Part print with two shaded views. Sizes in mm from the minimum x, y, z corner. A direction names the side the tool comes from. Coordinates: 2 decimals unless noted, no trailing zeros. Write each loop counter-clockwise with the first axis right and the second up, starting at its lowest first coordinate (ties: lowest second). Pieces come first, ordered by that corner, then holes.
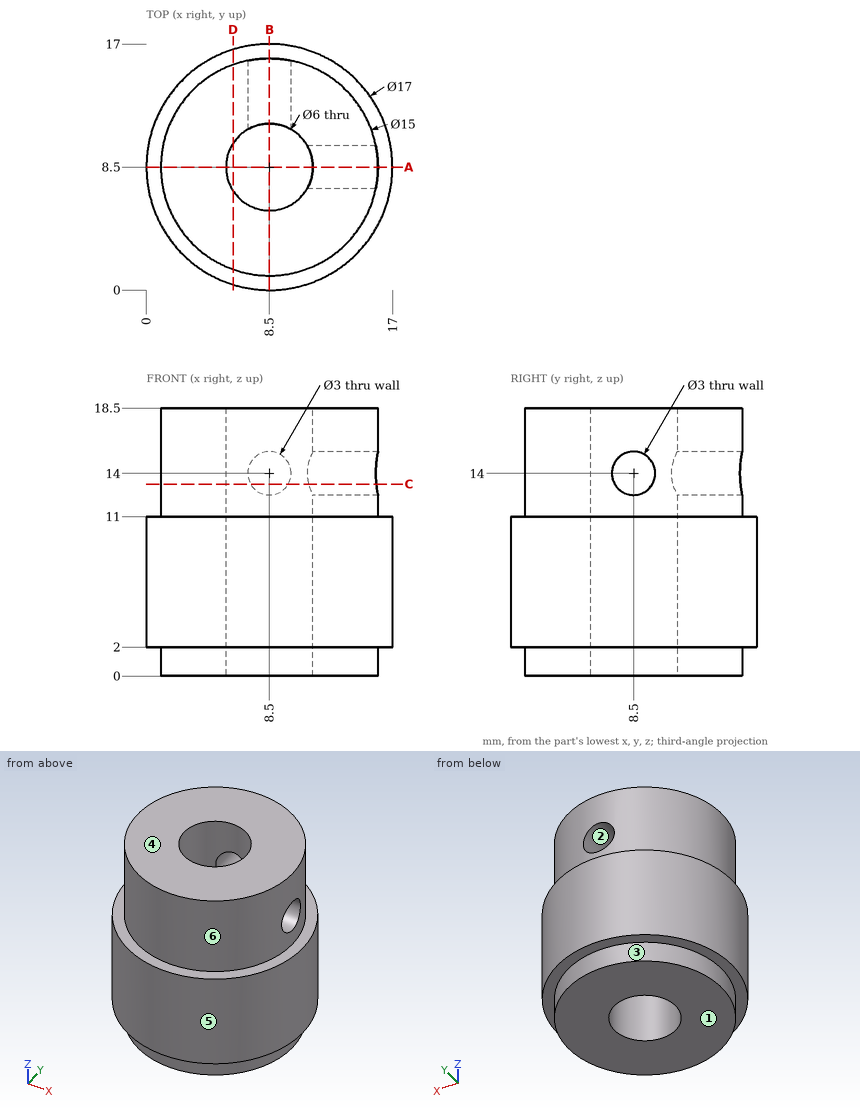
(1) Slice it at C-C, the plane z = 13.25. List the corners of the cut face in (x, y).
(2) Probe L1, parallel to Y at x = 8.5, z = 4.5; L2, parallel to Y at x = 8.5, z = 1.5; L3, parallel to X at y = 7.5, z = 11.5. List the from-to ranges inside material, lowest first.
(3) Slice it at A-A, the plane y = 8.5. List the corners of the cut face in (x, z).
(4) Flat gauge pins, fed straight in: P1, Ø1, axis at x = 4, z = 7, coming from the +Y side; P2, Ø2, axis at y = 15, z = 13, coming from the -X side; P3, Ø3.5, axis at y = 8.5, z = 14, coming from the -X side. Where does each tip first touch, or does it go through?
(5) Slice it at D-D, the plane x = 6. List the corners of the cut face in (y, z), and give its area (3 significant figures).
(6) 3-axis set-ups, long thin cutter, end or side, ignore diameter. For the marked faces 5 and 6: which of +Z, -Z, +X, -X, +Y, -Y reach the whole face in a straight line?
(7) Two-plate mould, pull along Z, no slides. Class the marked faces 1, 2, 3 and 4: pulls with the +Z half, pulls with the -Z half, needs draft (parallel to the pull), parting line crosses it, or undercut.
Results:
1. outline: (7.2, 11.2) - (7.2, 15.89) arc R7.5 ccw (long way) to (15.89, 7.2) - (11.2, 7.2) arc R3 cw (long way) to start; (9.8, 11.2) arc R3 cw to (11.2, 9.8) - (15.89, 9.8) arc R7.5 ccw to (9.8, 15.89) - close
2. L1: y = 0 to 5.5, 11.5 to 17
2. L2: y = 1 to 5.5, 11.5 to 16
2. L3: x = 1.07 to 5.67, 11.33 to 15.93
3. outline: (0, 2) - (1, 2) - (1, 0) - (5.5, 0) - (5.5, 18.5) - (1, 18.5) - (1, 11) - (0, 11) - close; (11.5, 0) - (16, 0) - (16, 2) - (17, 2) - (17, 11) - (16, 11) - (16, 12.5) - (11.5, 12.5) - close; (11.5, 15.5) - (16, 15.5) - (16, 18.5) - (11.5, 18.5) - close
4. P1: stops at y = 16
4. P2: stops at x = 3.4
4. P3: stops at x = 1
5. outline: (0.38, 2) - (1.43, 2) - (1.43, 0) - (6.84, 0) - (6.84, 18.5) - (1.43, 18.5) - (1.43, 11) - (0.38, 11) - close; (10.16, 0) - (15.57, 0) - (15.57, 2) - (16.62, 2) - (16.62, 11) - (15.57, 11) - (15.57, 18.5) - (10.16, 18.5) - close
5. area: 219 mm2
6. face 5: +Z, -Z
6. face 6: +Z
7. face 1: pulls with the -Z half
7. face 2: undercut
7. face 3: needs draft
7. face 4: pulls with the +Z half
